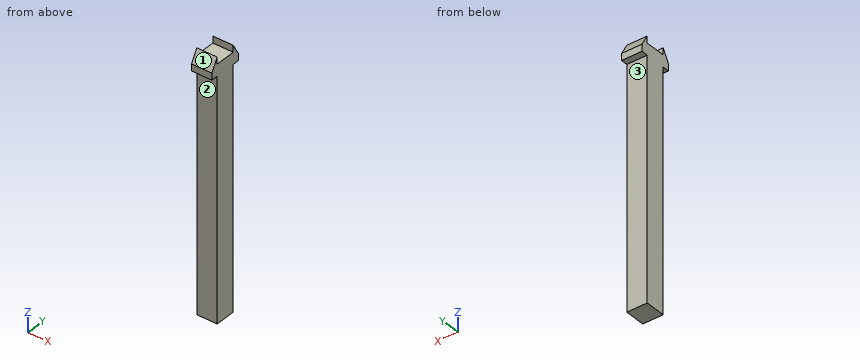
```python
from build123d import *

# Parameters (mm, degrees)
SKETCH1_W           = 15
SKETCH1_H           = 15
BOSS_EXTRUDE1_DEPTH = 190
BOSS_EXTRUDE2_DEPTH = 15
SKETCH3_W           = 15
SKETCH3_H           = 15
CUT_EXTRUDE1_DEPTH  = 5


with BuildPart() as part:
    # Sketch1 → Boss-Extrude1 (new body)
    with BuildSketch(Plane.XY):
        Rectangle(SKETCH1_W, SKETCH1_H)
    extrude(amount=BOSS_EXTRUDE1_DEPTH)

    # Sketch2 → Boss-Extrude2 (add)
    with BuildSketch(Plane.ZY.offset(7.5)):
        Polygon((190, 7.5), (181.339745962, 12.5), (176.339745962, 12.5), (176.339745962, 7.5), align=None)
        Polygon((176.339745962, -12.5), (176.339745962, -7.5), (190, -7.5), (181.339745962, -12.5), align=None)
    extrude(amount=-BOSS_EXTRUDE2_DEPTH)

    # Sketch3 → Cut-Extrude1 (cut)
    with BuildSketch(Plane.XY.offset(190)):
        Rectangle(SKETCH3_W, SKETCH3_H)
    extrude(amount=-CUT_EXTRUDE1_DEPTH, mode=Mode.SUBTRACT)


solid = part.part
```
Read the model definition and answer for the solid it produces. Units are mm, in the model's axes. Face numbers are marked on the shaded views. A direction names the side the tool comes from. Round coordinates to 2 decimals unless told otherwise and drop trailing zeros. Loops run counter-clockwise (first coordinate to the right, second up) from the corner with the lowest first, then second, coordinate; pieces in that order, holes last. Notation, with made-up numbers: (69, 50) -> (102, 50) arc R32 ccw to (102, 86) -> close; hole circle Ø1 at (12, -5.5). An arc over 180 degrees is marked (long way). One line per item, written item: value.
1) A cutting plane is placed at A-A (x = -3.5). Determine the outline of the cut face in (y, z), and give its area (3 significant figures).
Answer list:
outline: (-12.5, 176.34) -> (-7.5, 176.34) -> (-7.5, 0) -> (7.5, 0) -> (7.5, 176.34) -> (12.5, 176.34) -> (12.5, 181.34) -> (7.5, 190) -> (7.5, 185) -> (-7.5, 185) -> (-7.5, 190) -> (-12.5, 181.34) -> close
area: 2,870 mm²
2) Flat-ended cylindrical pins translate along their axes: P1, Ø5, axis at x = -5.5, z = 117.5, coming from the -Y side; P2, Ø4, axis at x = 0, z = 187, coming from the -Y side; P3, Ø3, axis at x = -2, z = 143, coming from the +Y side. Find the tip coordinate at first contact, or state that the pin passes through.
Answer list:
P1: stops at y = -7.5
P2: stops at y = -10.39
P3: stops at y = 7.5
3) For the marked faces 1, 2 and 3, determine the directions among +Z, -Z, +X, -X, +Y, -Y from which every point of the face is accessible in a straight line to the end or side of a thin tool.
Answer list:
face 1: +Z, +X, -X, -Y
face 2: -Z, +X, -X, -Y
face 3: -Z, +X, -X, +Y
4) A cutting plane is placed at C-C (z = 41.5). Determine the outline of the cut face in (x, y).
Answer list:
outline: (-7.5, -7.5) -> (7.5, -7.5) -> (7.5, 7.5) -> (-7.5, 7.5) -> close
5) A cutting plane is placed at B-B (y = 2.5). Determine the outline of the cut face in (x, z).
Answer list:
outline: (-7.5, 0) -> (7.5, 0) -> (7.5, 185) -> (-7.5, 185) -> close
6) Consider L1, parallel to Y at x = 0.25, z = 140; L2, parallel to Z at x = 3.5, y = -3; L3, parallel to Z at x = 0, y = 11.5. Determine where each line is inside the solid, lowest interval first. Write a range as [from, to].
Answer list:
L1: y = [-7.5, 7.5]
L2: z = [0, 185]
L3: z = [176.34, 183.07]
